Design review of the part built by this model. Coordinates are the model's own, in mm. Face numbers are marked on the shaded views. A direction names the side the tool comes from. Give positions to 0.01 mm unless a question says otherwise; leave off trailing zeros. Write each loop counter-clockwise with the first axis right and the second up, starting at its lowest first coordinate (ties: lowest second). Pieces come first, ordered by that corner, then holes. Notation, with made-up numbers: M -23.75,0 L -18.75,0 A31 cw -18.75,28 Z; hole C 59,51 d7. An arc over 180 degrees is marked long. Write each question's results on one line, items separated by ' | '. Start each with the question number.
Autodesk Inventor part; units mm, degrees
ref_plane "YZ Plane" through (0, 0, 0) normal (1, 0, 0) x (0, 1, 0)
ref_plane "XZ Plane" through (0, 0, 0) normal (0, 1, 0) x (-1, 0, 0)
ref_plane "XY Plane" through (0, 0, 0) normal (0, 0, 1) x (1, 0, 0)
sketch "Esquisse1" plane through (0, 0, 0) normal (0, 1, 0) x (-1, 0, 0)
  circle A0 centre (0, 0) radius 2.75
  dimension "d0" = 5.5
extrude "Extrusion1" add sketch "Esquisse1" along normal mid plane 10
sketch "Esquisse2" plane through (0, -5, 0) normal (0, -1, 0) x (1, 0, 0)
  circle A0 centre (0, 0) radius 2
  dimension "d3" = 4
extrude "Extrusion2" cut sketch "Esquisse2" against normal blind 5
fillet "Congé1" radius 0.5 1 edges at (2.75, 5, 0)
sketch "Esquisse3" plane through (0, -5, 0) normal (0, -1, 0) x (1, 0, 0)
  line L0 (9.7978, 4.7343) -> (6.189, 4.7343)
  line L1 (6.189, 4.7343) -> (6.189, -4.7343)
  line L2 (6.189, -4.7343) -> (9.7978, -4.7343)
  line L3 (9.7978, -4.7343) -> (9.7978, 4.7343)
  circle A0 centre (0, 0) radius 2.75
  line L4 (2.75, 0) -> (-2.75, 0) construction
  line L5 (9.7978, 0) -> (6.189, 0) construction
  line L6 (2.75, 3.5) -> (-2.75, 3.5)
  line L7 (-2.75, 3.5) -> (-2.75, -3.5)
  line L8 (-2.75, -3.5) -> (2.75, -3.5)
  line L9 (2.75, -3.5) -> (2.75, 3.5)
  line L10 (2.75, 0) -> (-2.75, 0) construction
  dimension "d7" = 5.5
  dimension "d8" = 5.5
  dimension "d9" = 7
extrude "Extrusion3" add sketch "Esquisse3" against normal blind 5 contours L9 L8 L7 A0 | A0 L7 L6 L9
equation "\"d8\" = d7"
properties part number "button"
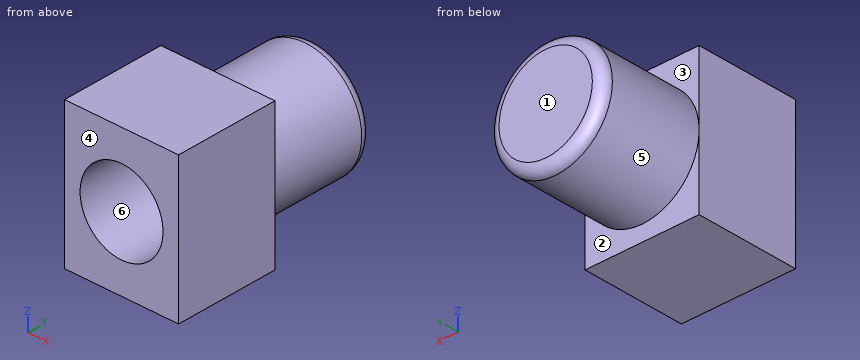
Q1. We need section A-A on x = 0. Write out the cut boundary in (y, z), and give its area (3 significant figures).
Q2. The part is to be moulded in two halves that separate along Z. For the marked faces 4, 5 and 6, say which applies: pulls with the +Z half, pulls with the -Z half, needs draft (parallel to the pull), parting line crosses it, or undercut.
Q3. We need section D-D on y = 1.75. Write out the cut boundary in (x, z), and give its area (3 significant figures).
Q4. We need section C-C on z = -3. Write out the cut boundary in (x, y), and give its area (3 significant figures).
Q5. We need section B-B on y = -3.5. Write out the cut boundary in (x, z), and give its area (3 significant figures).
Q6. For the marked faces 1, 2 and 3, list the 3-axis set-ups (+Z, -Z, +X, -X, +Y, -Y) from which the entire face can be reached by the end or side of a thin tool; tool diameter is ignored.
Q7. For pin 1 Ø1.2 at (x, z) = (0, -1) entering from -Y; pin 2 Ø4 at (y, z) = (2, 1.5) entering from -X; pin 3 Ø1.5 at (x, y) = (1.5, 3) entering from -Z, all flat-tipped, find the tip position at first contact; note any pin that passes through.
Q8. Wall thickness on line 1 along Z through (x, y) = (0, -1.75); line 2 along Y through (x, z) = (-1.2, 0.75); line 3 along X through (y, z) = (-1.5, -1.25): over which ranges is each line inside the solid? List them lowest first. Write a range as from..to.
Answer sheet:
1) outline: M -5,-3.5 L 0,-3.5 L 0,-2.75 L 4.5,-2.75 A0.5 ccw 5,-2.25 L 5,2.25 A0.5 ccw 4.5,2.75 L 0,2.75 L 0,3.5 L -5,3.5 L -5,2 L 0,2 L 0,-2 L -5,-2 Z | area: 42.4 mm^2
2) face 4: needs draft | face 5: parting line crosses it | face 6: undercut
3) outline: C 0,0 d5.5 | area: 23.8 mm^2
4) outline: M -2.75,-5 L 2.75,-5 L 2.75,0 L -2.75,0 Z | area: 27.5 mm^2
5) outline: M -2.75,-3.5 L 2.75,-3.5 L 2.75,3.5 L -2.75,3.5 Z; hole C 0,0 d4 | area: 25.9 mm^2
6) face 1: +Z, -Z, +X, -X, +Y | face 2: -Z, +Y | face 3: +Z, +Y
7) pin 1: y = 0 | pin 2: x = -2.75 | pin 3: z = -2.65
8) line 1: -3.5..-2, 2..3.5 | line 2: 0..5 | line 3: -2.75..-1.56, 1.56..2.75
